from build123d import *

# Parameters (mm, degrees)
SKETCH1_W           = 26.2
SKETCH1_H           = 26.2
SKETCH1_W_2         = 20.2
SKETCH1_H_2         = 20.2
BOSS_EXTRUDE1_DEPTH = 20
SKETCH2_R           = 4
BOSS_EXTRUDE4_DEPTH = 26.2


with BuildPart() as part:
    # Sketch1 → Boss-Extrude1 (new body)
    with BuildSketch(Plane(origin=(0, 0, 0), x_dir=(1, 0, 0), z_dir=(0, 1, 0))):
        with Locations((10.1, 10.1)):
            Rectangle(SKETCH1_W, SKETCH1_H)
        with Locations((10.1, 10.1)):
            Rectangle(SKETCH1_W_2, SKETCH1_H_2, mode=Mode.SUBTRACT)
    extrude(amount=BOSS_EXTRUDE1_DEPTH)

    # Sketch2 → Boss-Extrude4 (add)
    # profile 1 of 3: a face of its own
    with BuildSketch(Plane.XY.offset(3)):
        with BuildLine():
            ThreePointArc((34.3, 10), (33.279298444, 13.639778856), (30.514859965, 16.218092586))
            ThreePointArc((30.514859965, 16.218092586), (26.780404048, 16.980689081), (23.2, 15.673623181))
            Line((23.2, 15.673623181), (23.2, 4.326376819))
            ThreePointArc((23.2, 4.326376819), (26.780404048, 3.019310919), (30.514859965, 3.781907414))
            ThreePointArc((30.514859965, 3.781907414), (33.279298444, 6.360221144), (34.3, 10))
        make_face()
        with Locations((27.3, 10)):
            Circle(SKETCH2_R, mode=Mode.SUBTRACT)
    # profile 2 of 3: a face of its own
    with BuildSketch(Plane.XY.offset(3)):
        with BuildLine():
            Line((30.514859965, 16.218092586), (23.2, 20))
            Line((23.2, 20), (23.2, 15.673623181))
            ThreePointArc((23.2, 15.673623181), (26.780404048, 16.980689081), (30.514859965, 16.218092586))
        make_face()
    # profile 3 of 3: a face of its own
    with BuildSketch(Plane.XY.offset(3)):
        with BuildLine():
            ThreePointArc((30.514859965, 3.781907414), (26.780404048, 3.019310919), (23.2, 4.326376819))
            Line((23.2, 4.326376819), (23.2, 0))
            Line((23.2, 0), (30.514859965, 3.781907414))
        make_face()
    extrude(amount=-BOSS_EXTRUDE4_DEPTH)


solid = part.part
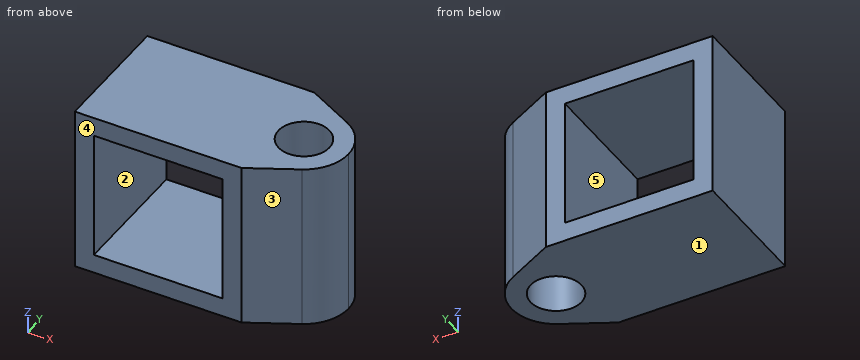
Check sheet for the modelled part. Datum: model origin and axes. Units: mm. Face numbers are marked on the shaded views. A direction names the side the tool comes from. Give positions to 0.01 mm unless a question says otherwise; leave off trailing zeros. Write each loop counter-clockwise with the first axis right and the second up, starting at its lowest first coordinate (ties: lowest second). Pieces come first, ordered by that corner, then holes. Notation, with made-up numbers: (11.25, 80.5) -> (28.25, 80.5) arc R26 ccw to (28.25, 99.5) -> close; hole circle Ø1 at (67.5, 48). An arc over 180 degrees is marked (long way). Use one line per item in the form item = value. Start each with the question number.
1. Section check B-B (x = 18). Record the cut outline in (y, z).
2. Thickness scan on line 1 along Z through (x, y) = (17, 15); line 2 along Y through (x, z) = (27.3, -7); line 3 along X through (y, z) = (7, 1). Record the ranges inside material, lowest first. Write a range as from..to.
3. Access from +Z, -Z, +X, -X, +Y, -Y to the whole of each face (thin tool, end or side, straight path). Record for the marked faces 4 and 5.
4. Section check D-D (y = 16.75). Record the cut outline in (x, z).
5. Go/stop test with flat-tipped pins: P1, Ø5, axis at x = 3, z = -15, coming from the -Y side; P2, Ø1, axis at y = 12.5, z = -9.5, coming from the +X side. Record where each tip stops, or that it passes through.
6. Mould release check, pull along Z, two halves, no side actions. Record for the marked faces 1, 2 and 3: pulls with the +Z half, pulls with the -Z half, needs draft (parallel to the pull), parting line crosses it, or undercut.
7. Section check A-A (z = -12.5). Record the cut outline in (x, y).
8. Section check C-C (y = 12.5). Record the cut outline in (x, z).
Conclusion:
q1.outline = (0, -23.2) -> (20, -23.2) -> (20, -20.2) -> (0, -20.2) -> close; (0, 0) -> (20, 0) -> (20, 3) -> (0, 3) -> close
q2.line_1 = -23.2..-20.2, 0..3
q2.line_2 = 2.12..6, 14..17.88
q2.line_3 = -3..24.65, 29.95..33.62
q3.face_4 = +Z, -Z, +X, -X, -Y
q3.face_5 = +Y, -Y
q4.outline = (-3, -23.2) -> (29.49, -23.2) -> (29.49, 3) -> (-3, 3) -> close; hole (0, -20.2) -> (20.2, -20.2) -> (20.2, 0) -> (0, 0) -> close
q5.P1 = through
q5.P2 = 34.01
q6.face_1 = pulls with the -Z half
q6.face_2 = undercut
q6.face_3 = needs draft
q7.outline = (-3, 0) -> (0, 0) -> (0, 20) -> (-3, 20) -> close; (20.2, 0) -> (23.2, 0) -> (30.51, 3.78) arc R7 ccw to (30.51, 16.22) -> (23.2, 20) -> (20.2, 20) -> close; hole circle Ø8 at (27.3, 10)
q8.outline = (-3, -23.2) -> (24.18, -23.2) -> (24.18, 3) -> (-3, 3) -> close; (30.42, -23.2) -> (33.84, -23.2) -> (33.84, 3) -> (30.42, 3) -> close; hole (0, -20.2) -> (20.2, -20.2) -> (20.2, 0) -> (0, 0) -> close
